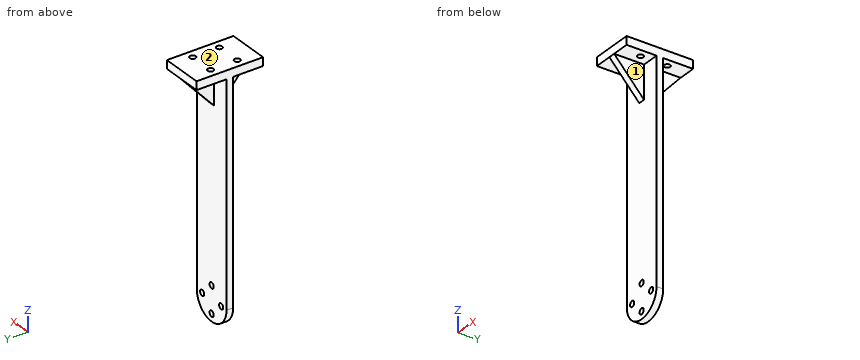
from build123d import *

# Parameters (mm, degrees)
BOSS_EXTRUDE1_DEPTH = 4
SKETCH2_W           = 25
SKETCH2_H           = 5
BOSS_EXTRUDE2_DEPTH = 17.95
SKETCH3_R           = 1.75
CUT_EXTRUDE1_DEPTH  = 6
SKETCH4_W           = 4
SKETCH4_H           = 17.95
BOSS_EXTRUDE3_DEPTH = 20
CUT_EXTRUDE2_DEPTH  = 15.5
SKETCH6_R           = 1.75
CUT_EXTRUDE3_DEPTH  = 22.95


with BuildPart() as part:
    # Sketch1 → Boss-Extrude1 (new body)
    with BuildSketch(Plane(origin=(0, 0, 0), x_dir=(1, 0, 0), z_dir=(0, 1, 0))):
        with BuildLine():
            Line((0, 0), (25, 0))
            Line((25, 0), (25, 136))
            ThreePointArc((25, 136), (12.5, 148.5), (0, 136))
            Line((0, 136), (0, 0))
        make_face()
    extrude(amount=BOSS_EXTRUDE1_DEPTH)

    # Sketch2 → Boss-Extrude2 (add)
    with BuildSketch(Plane(origin=(0, 4, 0), x_dir=(1, 0, 0), z_dir=(0, 1, 0))):
        with Locations((12.5, 2.5)):
            Rectangle(SKETCH2_W, SKETCH2_H)
    boss_extrude2 = extrude(amount=BOSS_EXTRUDE2_DEPTH)

    # Sketch3 → Cut-Extrude1 (cut, through all)
    with BuildSketch(Plane(origin=(0, 0, -5), x_dir=(-1, 0, 0), z_dir=(0, 0, -1))):
        with Locations((-20, 10)):
            Circle(SKETCH3_R)
        with Locations((-5, 10)):
            Circle(SKETCH3_R)
    cut_extrude1 = extrude(amount=-CUT_EXTRUDE1_DEPTH, mode=Mode.SUBTRACT)

    # Sketch4 → Boss-Extrude3 (add)
    with BuildSketch(Plane(origin=(0, 0, -5), x_dir=(-1, 0, 0), z_dir=(0, 0, -1))):
        with Locations((-12.5, 12.975)):
            Rectangle(SKETCH4_W, SKETCH4_H)
    boss_extrude3 = extrude(amount=BOSS_EXTRUDE3_DEPTH)

    # Sketch5 → Cut-Extrude2 (cut, through all)
    with BuildSketch(Plane(origin=(14.5, 0, 0), x_dir=(0, 0, -1), z_dir=(1, 0, 0))):
        Polygon((25, 4), (5, 21.95), (25, 21.95), align=None)
    cut_extrude2 = extrude(amount=-CUT_EXTRUDE2_DEPTH, mode=Mode.SUBTRACT)

    # Mirror1: Boss-Extrude2, Cut-Extrude1, Boss-Extrude3, Cut-Extrude2 across plane
    add(boss_extrude2.mirror(Plane.ZX.offset(2)))
    add(cut_extrude1.mirror(Plane.ZX.offset(2)), mode=Mode.SUBTRACT)
    add(boss_extrude3.mirror(Plane.ZX.offset(2)))
    add(cut_extrude2.mirror(Plane.ZX.offset(2)), mode=Mode.SUBTRACT)

    # Sketch6 → Cut-Extrude3 (cut, through all)
    with BuildSketch(Plane(origin=(0, 4, 0), x_dir=(1, 0, 0), z_dir=(0, 1, 0))):
        with Locations((12.5, 144)):
            Circle(SKETCH6_R)
        with Locations((20.5, 136)):
            Circle(SKETCH6_R)
        with Locations((12.5, 128)):
            Circle(SKETCH6_R)
        with Locations((4.5, 136)):
            Circle(SKETCH6_R)
    extrude(amount=-CUT_EXTRUDE3_DEPTH, mode=Mode.SUBTRACT)


solid = part.part
For this review, take the finished solid that the model builds, in its own axes (mm). Face numbers are marked on the shaded views. A direction names the side the tool comes from. Round coordinates to 2 decimals unless told otherwise and drop trailing zeros. Loops run counter-clockwise (first coordinate to the right, second up) from the corner with the lowest first, then second, coordinate; pieces in that order, holes last. Notation, with made-up numbers: (-12, -36.5) - (33, -36.5) arc R22 cw to (33, -20.5) - close; hole circle Ø4 at (26.5, 55). An arc over 180 degrees is marked (long way). One line per question, with ' | ' between items.
Q1. For pin 1 (19.5 mm diameter, centred on y = -6.5, z = -11.5, fed in from -X); pin 2 (4 mm diameter, centred on x = 20.5, z = -136, fed in from +Y); pin 3 (9 mm diameter, centred on y = 9, z = -16, fed in from -X); pin 4 (4 mm diameter, centred on x = 20, y = 10, fed in from -Z), all flat-tipped, find the tip position at first contact; note any pin that passes through.
Taken from the geometry:
pin 1: stops at x = 0 | pin 2: stops at y = 4 | pin 3: stops at x = 10.5 | pin 4: stops at z = -5
Q2. For line 1 along Y through (x, z) = (20, -1.45); line 2 along X through (y, z) = (-6, -3.7); line 3 along X through (y, z) = (2.6, -136), list the stretches that pass through material, from the lowest coordinate up. Write a range as [from, to].
Taken from the geometry:
line 1: y = [-17.95, -7.75], [-4.25, 8.25], [11.75, 21.95] | line 2: x = [0, 3.25], [6.75, 18.25], [21.75, 25] | line 3: x = [0, 2.75], [6.25, 18.75], [22.25, 25]
Q3. Take a section at D-D (y = -9.5). Give the boundary of the cut face in (x, z), and give its area (3 significant figures).
Taken from the geometry:
outline: (0, -5) - (10.5, -5) - (10.5, -14.42) - (14.5, -14.42) - (14.5, -5) - (25, -5) - (25, 0) - (0, 0) - close | area: 163 mm²
Q4. Take a section at A-A (z = -128). Give the boundary of the cut face in (x, y), and give its area (3 significant figures).
Taken from the geometry:
outline: (0, 0) - (10.75, 0) - (10.75, 4) - (0, 4) - close; (14.25, 0) - (25, 0) - (25, 4) - (14.25, 4) - close | area: 86.0 mm²
Q5. Take a section at B-B (x = 12.5). Give the boundary of the cut face in (y, z).
Taken from the geometry:
outline: (-17.95, -5) - (0, -25) - (0, -126.25) - (4, -126.25) - (4, -25) - (21.95, -5) - (21.95, 0) - (-17.95, 0) - close; (0, -148.5) - (4, -148.5) - (4, -145.75) - (0, -145.75) - close; (0, -142.25) - (4, -142.25) - (4, -129.75) - (0, -129.75) - close
Q6. Take a section at C-C (x = 4.5). Give the boundary of the cut face in (y, z), and give its area (3 significant figures).
Taken from the geometry:
outline: (-17.95, -5) - (-7.68, -5) - (-7.68, 0) - (-17.95, 0) - close; (-4.32, -5) - (0, -5) - (0, -134.25) - (4, -134.25) - (4, -5) - (8.32, -5) - (8.32, 0) - (-4.32, 0) - close; (0, -145.6) - (4, -145.6) - (4, -137.75) - (0, -137.75) - close; (11.68, -5) - (21.95, -5) - (21.95, 0) - (11.68, 0) - close | area: 714 mm²
Q7. Tool access review of the marked faces 1 and 2: name each direction out of +Z, -Z, +X, -X, +Y, -Y from which nothing blocks a thin tool from reaching the whole face with its end or side.
Taken from the geometry:
face 1: -Z, +X, -Y | face 2: +Z, +X, -X, +Y, -Y
